Study the drawing (mm; zero at the part's minimum x, y, z) and answer. Give positions to 0.01 mm unless a question says otherwise; leave off trailing zeros. Order: outer loops, then holes, each group sorted by start corner. A loop starts at its lowest first (then second) coordinate and runs counter-clockwise, first axis right, second up.
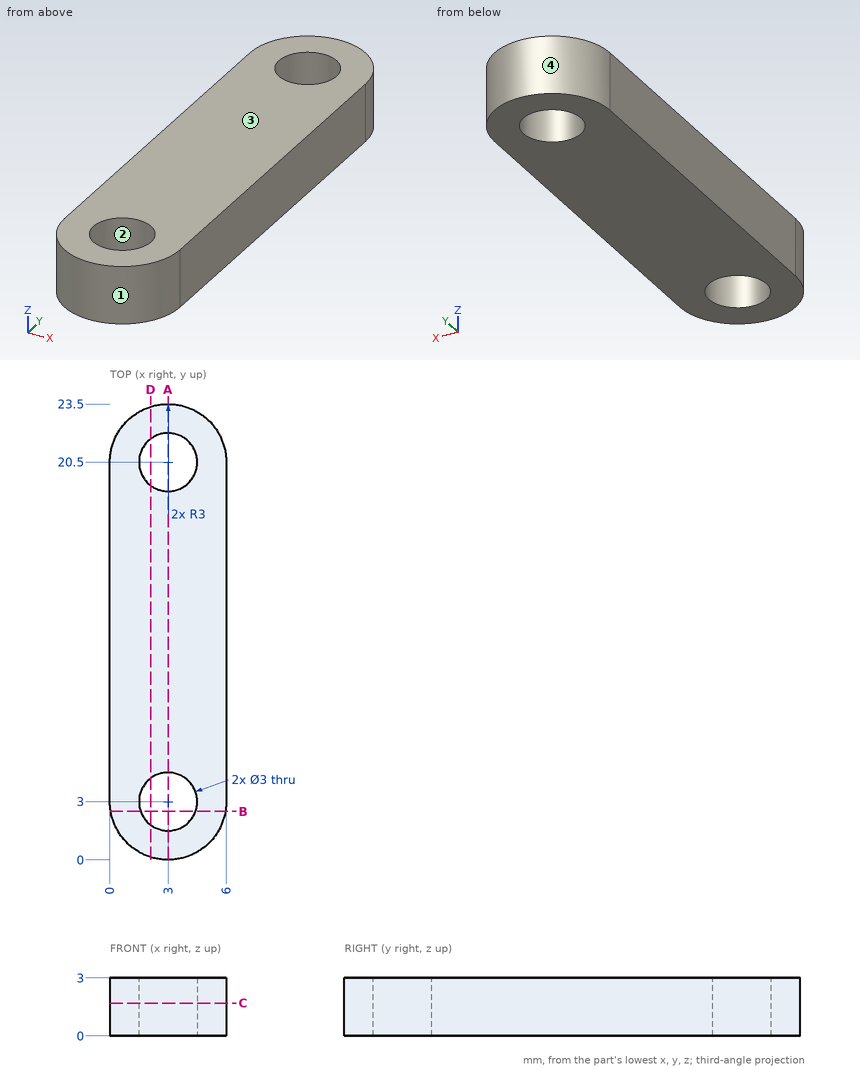
1) Find section B-B (y = 2.5). Write down the section's boundary in (x, z), then the cut area to 3 significant figures.
Geometry says:
outline: (0.04, 0) - (1.59, 0) - (1.59, 3) - (0.04, 3) - close; (4.41, 0) - (5.96, 0) - (5.96, 3) - (4.41, 3) - close
area: 9.26 mm2
2) Straight lines are drawn through the part: probe 1 along Y at (x, z) = (3, 2.05); probe 2 along Y at (x, z) = (2.5, 1.25); probe 3 along Y at (x, z) = (0.85, 1.8). For each, find the intervals that lie inside material, in ascending order.
Geometry says:
probe 1: y = 0 to 1.5, 4.5 to 19, 22 to 23.5
probe 2: y = 0.04 to 1.59, 4.41 to 19.09, 21.91 to 23.46
probe 3: y = 0.91 to 22.59
3) Find section C-C (z = 1.7). Write down the section's boundary in (x, y), then the cut area to 3 significant figures.
Geometry says:
outline: (0, 3) arc R3 ccw to (6, 3) - (6, 20.5) arc R3 ccw to (0, 20.5) - close; hole circle Ø3 at (3, 3); hole circle Ø3 at (3, 20.5)
area: 119 mm2
4) Find section D-D (x = 2.1). Write down the section's boundary in (y, z).
Geometry says:
outline: (0.14, 0) - (1.8, 0) - (1.8, 3) - (0.14, 3) - close; (4.2, 0) - (19.3, 0) - (19.3, 3) - (4.2, 3) - close; (21.7, 0) - (23.36, 0) - (23.36, 3) - (21.7, 3) - close
5) Given P1, Ø1, axis at x = 4, z = 2, coming from the +Y side, flat-ended and moving along its own axis, determine where the tip first touches the part or whether it passes through.
Geometry says:
P1: stops at y = 23.46
6) For a pull along Y with two mould halves and no side action, classify the marked faces 1, 2, 3 and 4 as +Y half, -Y half, draft (parallel to the pull), parting line (faces both ways), or undercut.
Geometry says:
face 1: -Y half
face 2: undercut
face 3: draft
face 4: +Y half
7) Find section A-A (x = 3). Write down the section's boundary in (y, z), then the cut area to 3 significant figures.
Geometry says:
outline: (0, 0) - (1.5, 0) - (1.5, 3) - (0, 3) - close; (4.5, 0) - (19, 0) - (19, 3) - (4.5, 3) - close; (22, 0) - (23.5, 0) - (23.5, 3) - (22, 3) - close
area: 52.5 mm2
